```python
from build123d import *
from build123d.topology import SkipClean

# Parameters (mm, degrees)
BOSS_EXTRUDE1_DEPTH  = 20
SKETCH3_R            = 1.25
SKETCH3_R_2          = 5
SKETCH3_R_3          = 2.25
CUT_EXTRUDE1_DEPTH   = 40
CUT_EXTRUDE2_DEPTH   = 40
MIRROR2_COPY_1_DEPTH = 40
BOSS_EXTRUDE3_DEPTH  = 2.5
SKETCH6_W            = 103.671116399
SKETCH6_H            = 23.957467505
CUT_EXTRUDE3_DEPTH   = 25
SKETCH7_W            = 105.212539013
SKETCH7_H            = 19.765490072
CUT_EXTRUDE4_DEPTH   = 25
SKETCH8_W            = 102.846794358
SKETCH8_H            = 18.402184695
CUT_EXTRUDE5_DEPTH   = 50
SKETCH9_W            = 100
SKETCH9_H            = 9.37939479
CUT_EXTRUDE6_DEPTH   = 50
FILLET2_R            = 10
FILLET3_R            = 400
FILLET4_START        = -2.563828285
FILLET4_DEPTH        = 5.127667015
FILLET4_START_2      = -10.0000001
FILLET4_2_DEPTH      = 20.0000001
FILLET4_START_3      = 19.9999999
FILLET4_3_DEPTH      = 163.0000001
SKETCH10_R           = 2
CUT_EXTRUDE7_DEPTH   = 10


with BuildPart() as part:
    # Sketch2 → Boss-Extrude1 (new, symmetric)
    with BuildSketch(Plane.XY):
        Polygon((0, 0), (200, 0), (200, 10), (-200, 10), (-200, 0), align=None)
    extrude(amount=BOSS_EXTRUDE1_DEPTH, both=True)

    # Sketch3 → Cut-Extrude1 (cut)
    with BuildSketch(Plane(origin=(0, 10, 0), x_dir=(1, 0, 0), z_dir=(0, 1, 0))):
        with Locations(Location((-4, 15.491933385, 0), (0, 0, 180))):
            Circle(SKETCH3_R)
        with Locations(Location((15.416407865, -4.281865077, 0), (0, 0, 180))):
            Circle(SKETCH3_R)
        with Locations(Location((-11.416407865, -11.210068308, 0), (0, 0, 180))):
            Circle(SKETCH3_R)
        with Locations(Location((0, 0, 0), (0, 0, 180))):
            Circle(SKETCH3_R_2)
        with Locations(Location((-190, 0, 0), (0, 0, 180))):
            Circle(SKETCH3_R_3)
        with Locations(Location((190, 0, 0), (0, 0, 270))):
            Circle(SKETCH3_R_3)
    extrude(amount=-CUT_EXTRUDE1_DEPTH, mode=Mode.SUBTRACT)

    # Sketch4 → Cut-Extrude2 (cut)
    with BuildSketch(Plane(origin=(0, 10, 0), x_dir=(1, 0, 0), z_dir=(0, 1, 0))):
        Polygon((-205.682411406, 30.266574236), (-25, 30.266574236), (-25, 20), (-200, 10), (-205.682411406, 10), align=None)
    cut_extrude2 = extrude(amount=-CUT_EXTRUDE2_DEPTH, mode=Mode.SUBTRACT)

    # Mirror1: Cut-Extrude2 across plane
    add(cut_extrude2.mirror(Plane(origin=(0, 0, 0), x_dir=(0, 0, 1), z_dir=(1, 0, 0))), mode=Mode.SUBTRACT)

    # Mirror2: Cut-Extrude2 across plane
    add(cut_extrude2.mirror(Plane.XY), mode=Mode.SUBTRACT)

    # Mirror2 copy 1 sketch → Mirror2 copy 1 (cut)
    with BuildSketch(Plane(origin=(0, 10, 0), x_dir=(-1, 0, 0), z_dir=(0, 1, 0))):
        Polygon((-205.682411406, 30.266574236), (-25, 30.266574236), (-25, 20), (-200, 10), (-205.682411406, 10), align=None)
    extrude(amount=-MIRROR2_COPY_1_DEPTH, mode=Mode.SUBTRACT)

    # Sketch5 → Boss-Extrude3 (add, symmetric)
    with BuildSketch(Plane.XY):
        Polygon((-181.848966048, 10), (-20, 10), (-130, 20), align=None)
    boss_extrude3 = extrude(amount=BOSS_EXTRUDE3_DEPTH, both=True)

    # Mirror3: Boss-Extrude3 across plane
    add(boss_extrude3.mirror(Plane(origin=(0, 0, 0), x_dir=(0, 0, 1), z_dir=(1, 0, 0))))

    # Sketch6 → Cut-Extrude3 (cut, symmetric)
    with BuildSketch(Plane.XY):
        with Locations((-151.594267329, 11.978733753)):
            Rectangle(SKETCH6_W, SKETCH6_H)
    extrude(amount=CUT_EXTRUDE3_DEPTH, both=True, mode=Mode.SUBTRACT)

    # Sketch7 → Cut-Extrude4 (cut, symmetric)
    with BuildSketch(Plane.XY):
        with Locations((-52.606269507, 14.882745036)):
            Rectangle(SKETCH7_W, SKETCH7_H)
    extrude(amount=CUT_EXTRUDE4_DEPTH, both=True, mode=Mode.SUBTRACT)

    # Sketch8 → Cut-Extrude5 (cut)
    with BuildSketch(Plane.XY):
        with Locations((-51.423397179, -0.639817385)):
            Rectangle(SKETCH8_W, SKETCH8_H)
    extrude(amount=-CUT_EXTRUDE5_DEPTH, mode=Mode.SUBTRACT)

    # Sketch9 → Cut-Extrude6 (cut)
    with BuildSketch(Plane.XY):
        with Locations((50, 0.310302605)):
            Rectangle(SKETCH9_W, SKETCH9_H)
    extrude(amount=-CUT_EXTRUDE6_DEPTH, mode=Mode.SUBTRACT)

    # Fillet2
    fillet2_edges = [part.edges().sort_by_distance(p)[0] for p in [
        (200, 5, -10),
        (200, 5, 10),
    ]]
    fillet(fillet2_edges, radius=FILLET2_R)

    # Fillet3
    # the kernel refuses this fillet: 400 mm, written as the material it takes off along each edge
    with BuildSketch(Plane(origin=(130, 20, 143.859110373), x_dir=(0.9819042977432754, -0.1893777972025378, 0), z_dir=(0, 0, -1))) as fillet3_piece_1:
        with BuildLine():
            CenterArc((56.676030542, 399.981263631), FILLET3_R, 253.889095702, 15.55633982)
            Line((-54.322969389, 15.690719883), (-56.542949388, 8.004909008))
            Line((-56.542949388, 8.004909008), (-2.219979999, -7.685810875))
            Line((-2.219979999, -7.685810875), (0, -8))
            ThreePointArc((0, -8), (26.402250284, -8), (52.727069969, -7.999625273))
            Line((52.727069969, -7.999625273), (52.804500568, 0))
        make_face()
    extrude(amount=287.718220747, mode=Mode.SUBTRACT)

    # Fillet4: read off the stored shape, not the designer's step
    # Fillet4 outline → Fillet4 (add)
    with SkipClean():  # the faces are left unmerged after this step: merging them gives an invalid solid
        with BuildSketch(Plane.XY.offset(FILLET4_START)):
            with BuildLine():
                ThreePointArc((181.84896605, 10), (127.934669494, 16.116857351), (73.688568923, 14.880778993))
                Line((73.688568923, 14.880778993), (20, 10))
                Line((20, 10), (181.84896605, 10))
            make_face()
        extrude(amount=FILLET4_DEPTH)

    # Fillet4 2 outline → Fillet4 2 (add)
    with BuildSketch(Plane.XY.offset(FILLET4_START_2)):
        with BuildLine():
            ThreePointArc((181.84896605, 10), (127.934669494, 16.116857351), (73.688568923, 14.880778993))
            Line((73.688568923, 14.880778993), (20, 10))
            Line((20, 10), (181.84896605, 10))
        make_face()
    extrude(amount=FILLET4_2_DEPTH)

    # Fillet4 3 outline → Fillet4 3 (cut)
    with BuildSketch(Plane.YZ.offset(FILLET4_START_3)):
        with BuildLine():
            ThreePointArc((16.523566776, -2.5638331), (11.862037195, -5.053953558), (10, -10))
            Line((10, -10), (18, -10.0000001))
            Line((18, -10.0000001), (18, -2.369964609))
            Line((18, -2.369964609), (16.523566776, -2.5638331))
        make_face()
        with BuildLine():
            Line((16.523565368, 2.563833285), (18, 2.369964325))
            Line((18, 2.369964325), (18, 10))
            Line((18, 10), (10, 10))
            ThreePointArc((10, 10), (11.862036727, 5.053954091), (16.523565368, 2.563833285))
        make_face()
    extrude(amount=FILLET4_3_DEPTH, mode=Mode.SUBTRACT)

    # Sketch10 → Cut-Extrude7 (cut)
    with BuildSketch(Plane(origin=(0, 10, 0), x_dir=(1, 0, 0), z_dir=(0, 1, 0))):
        with Locations(Location((80, 13.351433229, 0), (0, 0, 180))):
            Circle(SKETCH10_R)
        with Locations(Location((-80, -13.351433229, 0), (0, 0, 180))):
            Circle(SKETCH10_R)
    extrude(amount=-CUT_EXTRUDE7_DEPTH, mode=Mode.SUBTRACT)


solid = part.part
```
For this review, take the finished solid that the model builds, in its own axes (mm). A direction names the side the tool comes from. Round coordinates to 2 decimals unless told otherwise and drop trailing zeros. Loops run counter-clockwise (first coordinate to the right, second up) from the corner with the lowest first, then second, coordinate; pieces in that order, holes last.
(1) Clearance check with flat-ended pins moving along their axes: P1, Ø1.5, axis at y = 2.5, z = -8, coming from the -X side; P2, Ø12, axis at x = -13, z = 11.5, coming from the -Y side; P3, Ø9, axis at x = 0, z = 0, coming from the +Y side; P4, Ø3, axis at x = -11.42, z = 11.21, coming from the +Y side. State where each tip first meets the part, or that it passes through.
Returned:
P1: stops at x = 100
P2: stops at y = 0
P3: passes through
P4: stops at y = 5
(2) Wall thickness on line 1 along Z through (x, y) = (190, 5.5); line 2 along Z through (x, y) = (24, 1); line 3 along Y through (x, z) = (47.5, 10): over which ranges is each line inside the solid? List them lowest first.
Returned:
line 1: z = -10.57 to -2.25, 2.25 to 10.57
line 2: z = 0 to 20
line 3: y = 0 to 10
(3) We need section A-A (x = 70). Give the boundary of the cut face in (y, z), plus the area to 3 significant figures.
Returned:
outline: (0, 0) - (5, 0) - (5, -17.43) - (10, -17.43) - (10, -10) arc R7.5 cw to (14.55, -3.11) - (14.55, 3.11) arc R7.5 cw to (10, 10) - (10, 17.43) - (0, 17.43) - close
area: 307 mm2
(4) We need section C-C (x = -20.5). Give the boundary of the cut face in (y, z), plus the area to 3 significant figures.
Returned:
outline: (0, 0) - (5, 0) - (5, 20) - (0, 20) - close
area: 100 mm2
(5) We need section B-B (x = 36). Give the boundary of the cut face in (y, z), plus the area to 3 significant figures.
Returned:
outline: (0, 0) - (5, 0) - (5, -19.37) - (10, -19.37) - (10, -10) arc R7.5 cw to (11.45, -5.56) - (11.45, 5.56) arc R7.5 cw to (10, 10) - (10, 19.37) - (0, 19.37) - close
area: 311 mm2
(6) Mouldability with a two-part tool opening along X and no side actions: class faces 1 (the flat face through (-61.856, 2.535, 17.894)), 2 (the cylindrical face through (3, 5, 4)), 3 (the flat face through (78.2, 10, 10.5)), 4 (the flat face through (125.023, 6.181, -14.284)) as released by +X, released by -X, zero draft, split by the parting line, or undercut.
Returned:
face 1: released by -X
face 2: undercut
face 3: zero draft
face 4: released by +X
(7) Tool access review of faces 5 (the flat face through (0, 7, -12)), 6 (the flat face through (-53, 3, 0)), 7 (the flat face through (52, 3, 0)), 8 (the flat face through (-51, 5, 10)): name each direction out of +Z, -Z, +X, -X, +Y, -Y from which nothing blocks a thin tool from reaching the whole face with its end or side.
Returned:
face 5: +Z, -Z, -X, +Y, -Y
face 6: -Z, -X, +Y, -Y
face 7: -Z, -X, -Y
face 8: +Z, -Z, -X, +Y
